from build123d import *

# Parameters (mm, degrees)
F0_W     = 16
F0_H     = 27
F0_R     = 1.1
F1_DEPTH = 1.47957
F3_W     = 3.8
F3_H     = 6
F4_DEPTH = 10
F3_W_2   = 4.992
F5_DEPTH = 1.85


with BuildPart() as f1:
    # F0 (on Front) → F1 (new body)
    with BuildSketch(Plane.XZ):
        with Locations((8, -13.5)):
            Rectangle(F0_W, F0_H)
        with Locations((3, -23.75)):
            Circle(F0_R, mode=Mode.SUBTRACT)
        with Locations((13, -23.75)):
            Circle(F0_R, mode=Mode.SUBTRACT)
    extrude(amount=F1_DEPTH)

    # F3 (on face) → F4 (join)
    with BuildSketch(Plane.XZ.offset(1.47957)):
        with Locations((3.604, -3)):
            Rectangle(F3_W, F3_H)
        with Locations((12.396, -3)):
            Rectangle(F3_W, F3_H)
    extrude(amount=F4_DEPTH)

    # F3 (on face) → F5 (join)
    with BuildSketch(Plane.XZ.offset(1.47957)):
        with Locations((8, -3)):
            Rectangle(F3_W_2, F3_H)
    extrude(amount=F5_DEPTH)


solid = f1.part
Work out the finished part from the listing and answer in its coordinate system (mm). A direction names the side the tool comes from. Round coordinates to 2 decimals unless told otherwise and drop trailing zeros. Order: outer loops, then holes, each group sorted by start corner. A loop starts at its lowest first (then second) coordinate and runs counter-clockwise, first axis right, second up. Notation, with made-up numbers: M -14.5,-24.75 L 38.5,-24.75 A32 cw 38.5,6.25 Z; hole C 28.25,64 d9. An arc over 180 degrees is marked long. One line per item, written item: value.
Q1. Flat-ended cylindrical pins translate along their axes: pin 1 (3 mm diameter, centred on y = -6.5, z = -4, fed in from +X); pin 2 (2.5 mm diameter, centred on x = 3, z = -23.75, fed in from -Y); pin 3 (3 mm diameter, centred on x = 8.5, y = -6.5, fed in from -Z); pin 4 (1.8 mm diameter, centred on y = -8, z = -2, fed in from -X). Find the tip coordinate at first contact, or state that the pin passes through.
Derived:
pin 1: x = 14.3
pin 2: y = -1.48
pin 3: through
pin 4: x = 1.7
Q2. For faces 1 (the face through (10.496, -7, -3)), 2 (the face through (1.704, -6, -3)), 3 (the face through (11, -6, -6)), determine the directions among +Z, -Z, +X, -X, +Y, -Y from which every point of the face is accessible in a straight line to the end or side of a thin tool.
Derived:
face 1: +Z, -Z, -Y
face 2: +Z, -Z, -X, -Y
face 3: -Z, +X, -X, -Y
Q3. Find section C-C on y = -5.5. Write down the section's boundary in (x, z).
Derived:
outline: M 1.7,-6 L 5.5,-6 L 5.5,0 L 1.7,0 Z; M 10.5,-6 L 14.3,-6 L 14.3,0 L 10.5,0 Z
Q4. Straight lines are drawn through the part: line 1 (X direction, y = -10, z = -1.75); line 2 (Z direction, x = 13, y = -0.5); line 3 (Z direction, x = 5.75, y = -2). For each, find the intervals that lie inside material, in ascending order.
Derived:
line 1: 1.7 to 5.5, 10.5 to 14.3
line 2: -27 to -24.85, -22.65 to 0
line 3: -6 to 0
Q5. Find section A-A on z = -23.75. Write down the section's boundary in (x, y).
Derived:
outline: M 0,-1.48 L 1.9,-1.48 L 1.9,0 L 0,0 Z; M 4.1,-1.48 L 11.9,-1.48 L 11.9,0 L 4.1,0 Z; M 14.1,-1.48 L 16,-1.48 L 16,0 L 14.1,0 Z
Q6. Find section B-B on x = 13. Write down the section's boundary in (y, z), then the cut area to 3 significant figures.
Derived:
outline: M -11.48,-6 L -1.48,-6 L -1.48,-22.65 L 0,-22.65 L 0,0 L -11.48,0 Z; M -1.48,-27 L 0,-27 L 0,-24.85 L -1.48,-24.85 Z
area: 96.7 mm²
Q7. Determine the mould class of faces 4 (the face through (8, 0, -13)), 5 (the face through (5.504, -7, -3)), 6 (the face through (14.296, -6, -3)) for opening direction X: released by +X, released by -X, zero draft, split by the parting line, or undercut.
Derived:
face 4: zero draft
face 5: undercut
face 6: released by +X
Q8. Find section D-D on y = -0.5. Write down the section's boundary in (x, z).
Derived:
outline: M 0,-27 L 16,-27 L 16,0 L 0,0 Z; hole C 3,-23.75 d2.2; hole C 13,-23.75 d2.2
